from build123d import *

# Parameters (mm, degrees)
SKETCH1_W           = 1249.2
SKETCH1_H           = 350
SKETCH1_W_2         = 1198.4
SKETCH1_H_2         = 299.2
BOSS_EXTRUDE1_DEPTH = 25.4
SKETCH2_R           = 4
CUT_EXTRUDE3_DEPTH  = 25.4
SKETCH3_R           = 4
CUT_EXTRUDE10_DEPTH = 5341.4


with BuildPart() as part:
    # Sketch1 → Boss-Extrude1 (new body)
    with BuildSketch(Plane.XY):
        with Locations((624.6, -175)):
            Rectangle(SKETCH1_W, SKETCH1_H)
        with Locations((624.6, -175)):
            Rectangle(SKETCH1_W_2, SKETCH1_H_2, mode=Mode.SUBTRACT)
    extrude(amount=-BOSS_EXTRUDE1_DEPTH)

    # Sketch2 → Cut-Extrude3 (cut)
    with BuildSketch(Plane(origin=(0, 0, 0), x_dir=(1, 0, 0), z_dir=(0, 1, 0))):
        with Locations(Location((325, 12.7, 0), (0, 0, 270))):
            Circle(SKETCH2_R)
        with Locations(Location((975.054095101, 12.7, 0), (0, 0, 270))):
            Circle(SKETCH2_R)
    extrude(amount=-CUT_EXTRUDE3_DEPTH, mode=Mode.SUBTRACT)

    # Sketch3 → Cut-Extrude10 (cut)
    with BuildSketch(Plane(origin=(0, 0, 0), x_dir=(0, 0, -1), z_dir=(1, 0, 0))):
        with Locations(Location((12.7, -100, 0), (0, 0, 180))):
            Circle(SKETCH3_R)
        with Locations(Location((12.7, -250, 0), (0, 0, 180))):
            Circle(SKETCH3_R)
    extrude(amount=CUT_EXTRUDE10_DEPTH, mode=Mode.SUBTRACT)


solid = part.part
Read the model definition and answer for the solid it produces. Units are mm, in the model's axes. A direction names the side the tool comes from. Give positions to 0.01 mm unless a question says otherwise; leave off trailing zeros. Write each loop counter-clockwise with the first axis right and the second up, starting at its lowest first coordinate (ties: lowest second). Pieces come first, ordered by that corner, then holes. Notation, with made-up numbers: (54, -37) - (61, -37) arc R20 cw to (61, -28) - close; hole circle Ø6 at (24.25, 40). An arc over 180 degrees is marked (long way). Use CSV: the item, a comma, the result in double quotes. Start each with the question number.
(1) Find section A-A (z = -12.7). Count the separate pieces of the cut face and the enclosed holes in it, plus the area to 3 significant figures.
(2) Consider line 1 along Y through (x, z) = (1239, -12.7); line 2 along X through (y, z) = (-311.5, -11.5); line 3 along Z through (x, y) = (325, -19). Determine where each line is inside the solid, lowest interval first.
(3) Find section C-C (x = 835). Give the vertices of the cut face in (y, z).
(4) For faces 5 (the flat face through (1223.8, -177, -13)), 6 (the flat face through (529, -330, 0)), determine the directions among +Z, -Z, +X, -X, +Y, -Y from which every point of the face is accessible in a straight line to the end or side of a thin tool.
(5) Determine the mould class of faces 1 (the flat face through (616, 0, -13)), 2 (the flat face through (0, -177, -13)), 3 (the flat face through (616, -350, -13)), 4 (the flat face through (616, -25.4, -13)) for opening direction Y: +Y half, -Y half, draft (parallel to the pull), parting line (faces both ways), or undercut.
(6) Find section B-B (y = -292). Give the vertices of the cut face in (x, z).
Findings below:
1,separate pieces,"6"
1,enclosed holes,"0"
1,area,"77,400 mm2"
2,line 1,"-350 to -254, -246 to -104, -96 to 0"
2,line 2,"0 to 25.4, 1223.8 to 1249.2"
2,line 3,"-25.4 to -16.7, -8.7 to 0"
3,outline,"(-350, -25.4) - (-324.6, -25.4) - (-324.6, 0) - (-350, 0) - close; (-25.4, -25.4) - (0, -25.4) - (0, 0) - (-25.4, 0) - close"
4,face 5,"+Z, -Z"
4,face 6,"+Z, +X, -X, +Y, -Y"
5,face 1,"+Y half"
5,face 2,"draft"
5,face 3,"-Y half"
5,face 4,"undercut"
6,outline,"(0, -25.4) - (25.4, -25.4) - (25.4, 0) - (0, 0) - close; (1223.8, -25.4) - (1249.2, -25.4) - (1249.2, 0) - (1223.8, 0) - close"
